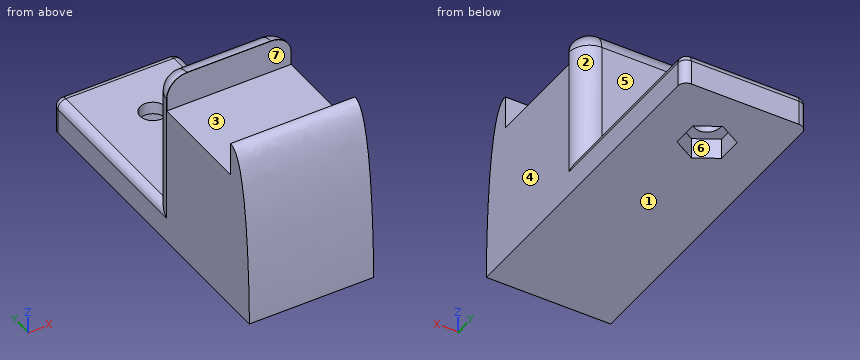
from build123d import *

# Parameters (mm, degrees)
PAD002_DEPTH    = 30
SKETCH009_R     = 3.1
POCKET004_DEPTH = 8.001
POCKET005_DEPTH = 5
FILLET005_R     = 4.9
FILLET006_R     = 4.9
FILLET007_R     = 2


with BuildPart() as part:
    # Sketch008 → Pad002 (new body)
    with BuildSketch(Plane.YZ):
        with BuildLine():
            add(Edge.make_bspline(
                [(-12.5, 42), (-20, 43), (-20, 0), (-20, 0)],
                knots=[0, 0, 0, 0, 1, 1, 1, 1], degree=3))
            Line((-20, 0), (57.5, 0))
            Line((57.5, 0), (57.5, 8))
            Line((57.5, 8), (17.5, 8))
            Line((17.5, 8), (17.5, 42))
            Line((17.5, 42), (12.5, 42))
            Line((12.5, 42), (12.5, 34))
            Line((12.5, 34), (-12.5, 34))
            Line((-12.5, 34), (-12.5, 42))
        make_face()
    extrude(amount=PAD002_DEPTH)

    # Sketch009 (on Face4 of Pad002) → Pocket004 (cut, through all)
    with BuildSketch(Plane(origin=(0, 0, 8), x_dir=(0, -1, 0), z_dir=(0, 0, 1))):
        with Locations((-42.5, 15)):
            Circle(SKETCH009_R)
    extrude(amount=-POCKET004_DEPTH, mode=Mode.SUBTRACT)

    # Sketch010 (on Face3 of Pocket004) → Pocket005 (cut)
    with BuildSketch(Plane.YX):
        Polygon((48.7, 14.99998), (45.600017, 20.369348), (39.400017, 20.369367), (36.3, 15.00002), (39.399983, 9.630652), (45.599983, 9.630633), align=None)
    extrude(amount=-POCKET005_DEPTH, mode=Mode.SUBTRACT)

    # Fillet005
    fillet005_edges = [part.edges().sort_by_distance(p)[0] for p in [
        (30, 17.5, 25),
        (0, 17.5, 25),
    ]]
    fillet(fillet005_edges, radius=FILLET005_R)

    # Fillet006
    fillet006_edges = [part.edges().sort_by_distance(p)[0] for p in [
        (15, 17.5, 42),
    ]]
    fillet(fillet006_edges, radius=FILLET006_R)

    # Fillet007
    fillet007_edges = [part.edges().sort_by_distance(p)[0] for p in [
        (15, 57.5, 8),
        (0, 37.5, 8),
        (30, 37.5, 8),
        (30, 57.5, 4),
        (0, 57.5, 4),
    ]]
    fillet(fillet007_edges, radius=FILLET007_R)


with BuildPart() as part_1:
    # Body005 placement: moved
    add(part.part.moved(Location((-660.5, 0, 0))))


solid = part_1.part
CAD build for the part. Positions are in the model's coordinates, mm. Face numbers are marked on the shaded views. A direction names the side the tool comes from. Coordinates: 2 decimals unless noted, no trailing zeros. Loops run counter-clockwise (first coordinate to the right, second up) from the corner with the lowest first, then second, coordinate; pieces in that order, holes last. Notation, with made-up numbers: (83.25, 41.5) -> (88.25, 41.5) arc R12 ccw to (88.25, 53.5) -> close; hole circle Ø1 at (21, 85). An arc over 180 degrees is marked (long way). One line per item, written item: value.
1. Pull direction Y, two halves, no side cores. Call the marked faces 4, 5, 6 and 7: pulls with the +Y half, pulls with the -Y half, needs draft (parallel to the pull), parting line crosses it, or undercut.
Answers:
face 4: needs draft
face 5: pulls with the +Y half
face 6: undercut
face 7: undercut
2. Which spindle directions (+Z, -Z, +X, -X, +Y, -Y) get a long thin tool onto all of the face, cutting with end or side? Do the marked faces 1, 2 and 3. Say none if no direction does.
Answers:
face 1: -Z, +X, -X, +Y, -Y
face 2: +Z, +X, +Y
face 3: +Z, +X, -X
3. Drill centre lines: line 1 (X direction, y = 42.5, z = 5.85); line 2 (Z direction, x = -642, y = 39.5); line 3 (Z direction, x = -647, y = 35). Where is each one in solid material? Low to high. Write a range as [from, to].
Answers:
line 1: x = [-660.5, -648.6], [-642.4, -630.5]
line 2: z = [5, 8]
line 3: z = [0, 8]
4. Slice it at A-A on y = 42.5. Write the cut outline in (x, z).
Answers:
outline: (-660.5, 0) -> (-650.87, 0) -> (-650.87, 5) -> (-648.6, 5) -> (-648.6, 8) -> (-658.5, 8) arc R2 ccw to (-660.5, 6) -> close; (-642.4, 5) -> (-640.13, 5) -> (-640.13, 0) -> (-630.5, 0) -> (-630.5, 6) arc R2 ccw to (-632.5, 8) -> (-642.4, 8) -> close
5. Slice it at B-B on y = 6. Write the cut outline in (x, z).
Answers:
outline: (-660.5, 0) -> (-630.5, 0) -> (-630.5, 34) -> (-660.5, 34) -> close
6. Flat gauge pins, fed straight in: P1, Ø4, axis at x = -653, z = 27, coming from the -Y side; P2, Ø5.5, axis at x = -644, y = 40.5, coming from the -Z side; P3, Ø12, axis at x = -636.5, z = 12.5, coming from the +Y side. Where does each tip first touch, or does it go through?
Answers:
P1: stops at y = -18.7
P2: stops at z = 5
P3: stops at y = 57.44
